from build123d import *

# Parameters (mm, degrees)
F0_R     = 12.7
F1_DEPTH = 30.1625
F2_W     = 28.956
F2_H     = 22.3266
F2_R     = 6.35
F3_DEPTH = 44.705
F5_DEPTH = 19.05
F7_DEPTH = 19.05
F8_R     = 3.302
F9_R     = 7.874
F10_R    = 3.302
F11_R    = 5.08


with BuildPart() as f1:
    # F0 (on Front) → F1 (new body, symmetric)
    with BuildSketch(Plane.XZ):
        with BuildLine():
            Line((-85.9282, -11.176), (108.2802, -11.176))
            Line((108.2802, -11.176), (108.2802, 11.176))
            Line((108.2802, 11.176), (-63.5762, 11.176))
            ThreePointArc((-63.5762, 11.176), (-101.733451, 26.981251), (-85.9282, -11.176))
        make_face()
        with Locations((-85.9282, 11.176)):
            Circle(F0_R, mode=Mode.SUBTRACT)
    extrude(amount=F1_DEPTH, both=True)

    # F2 (on face) → F3 (cut, through all)
    with BuildSketch(Plane(origin=(0, 0, -11.176), x_dir=(1, 0, 0), z_dir=(0, 0, -1))):
        with Locations((-100.4062, 0)):
            Rectangle(F2_W, F2_H)
        with Locations((69.4182, -7.8105)):
            Circle(F2_R)
        with Locations((-71.4502, 0)):
            Rectangle(F2_W, F2_H)
    extrude(amount=-F3_DEPTH, mode=Mode.SUBTRACT)

    # F4 (on face) → F5 (cut)
    with BuildSketch(Plane.XZ.offset(30.1625)):
        Polygon((31.3182, -11.176), (31.3182, 11.176), (-0.0762, 11.176), (5.9182, -11.176), align=None)
    extrude(amount=-F5_DEPTH, mode=Mode.SUBTRACT)

    # F6 (on face) → F7 (join)
    with BuildSketch(Plane.XZ.offset(30.1625)):
        with BuildLine():
            Line((31.3182, 9.144), (45.1104, 9.144))
            Line((45.1104, 9.144), (64.1604, 9.144))
            Line((64.1604, 9.144), (64.1604, 45.974))
            Line((64.1604, 45.974), (45.1104, 45.974))
            ThreePointArc((45.1104, 45.974), (41.536215, 27.258358), (31.3182, 11.176))
            Line((31.3182, 11.176), (31.3182, 9.144))
        make_face()
    extrude(amount=-F7_DEPTH)

    # F8
    f8_edges = [f1.edges().sort_by_distance(p)[0] for p in [
        (-63.5762, -20.6629, 11.176),
        (-63.5762, 20.6629, 11.176),
    ]]
    fillet(f8_edges, radius=F8_R)

    # F9
    f9_edges = [f1.edges().sort_by_distance(p)[0] for p in [
        (108.2802, 0, 11.176),
    ]]
    fillet(f9_edges, radius=F9_R)

    # F10
    f10_edges = [f1.edges().sort_by_distance(p)[0] for p in [
        (64.1604, -20.6375, 11.176),
    ]]
    fillet(f10_edges, radius=F10_R)

    # F11
    f11_edges = [f1.edges().sort_by_distance(p)[0] for p in [
        (64.1604, -20.6375, 45.974),
    ]]
    fillet(f11_edges, radius=F11_R)


solid = f1.part
Source: CAD feature listing. Evaluate the final solid. Frame: model axes, mm. A direction names the side the tool comes from. Give positions to 0.01 mm unless a question says otherwise; leave off trailing zeros. Write each loop counter-clockwise with the first axis right and the second up, starting at its lowest first coordinate (ties: lowest second). Pieces come first, ordered by that corner, then holes. Notation, with made-up numbers: M 27.25,21 L 60.25,21 A21 cw 60.25,32 Z; hole C 9,-8 d3. An arc over 180 degrees is marked long. Return JSON: item names as keys, results as strings. Group by question number.
1) Draft query along X for faces 1 (the face through (31.318, -21, 0)), 2 (the face through (15, -11.112, 0)), 3 (the face through (64.16, -21, 28)), 4 (the face through (-102.2, 20.5, 26.5)). Return one class per face: released by +X, released by -X, zero draft, split by the parting line, or undercut.
2) Cut plane B-B, the plane z = 17.5. Output: boundary loops of the cut face in (x, y), then the cut area to 3 significant figures.
3) Cut plane D-D, the plane y = 4. Output: boundary loops of the cut face in (x, z), then the cut area to 3 significant figures.
4) Set-up query: faces 5 (the face through (21, 6, 11.176)), 6 (the face through (-56.972, 0, 0)), 7 (the face through (53, -11.112, 29)). Return all of +Z, -Z, +X, -X, +Y, -Y with unobstructed straight access to the full face (end or side cutting, diameter ignored); none if empty.
5) First-contact query: pin 1 Ø5 at (y, z) = (11.5, 15.5) entering from -X; pin 2 Ø1.5 at (x, y) = (-25.5, 3) entering from +Z; pin 3 Ø18 at (y, z) = (-2, -4.5) entering from -X. Flat tips, straight axial feed; report the tip coordinate or a pass-through.
6) Ray query, L1, parallel to Y at x = -92.5, z = -4; L2, parallel to X at y = -15, z = -0.5; L3, parallel to Z at x = 50.5, y = 16. Return the intervals inside material, ascending.
7) Cut plane A-A, the plane y = 23. Output: boundary loops of the cut face in (x, z).
8) Cut plane C-C, the plane x = 49.5. Output: boundary loops of the cut face in (y, z), then the cut area to 3 significant figures.
Data:
{
 "1": {"face 1": "undercut", "face 2": "undercut", "face 3": "released by +X", "face 4": "split by the parting line"},
 "2": {"outline": "M -107.37,-30.16 L -96.94,-30.16 L -96.94,-11.16 L -107.37,-11.16 Z; M -107.37,11.16 L -96.94,11.16 L -96.94,30.16 L -107.37,30.16 Z; M -74.91,-30.16 L -64.49,-30.16 L -64.49,-11.16 L -74.91,-11.16 Z; M -74.91,11.16 L -64.49,11.16 L -64.49,30.16 L -74.91,30.16 Z; M 36.38,-30.16 L 64.16,-30.16 L 64.16,-11.11 L 36.38,-11.11 Z", "area": "1,320 mm²"},
 "3": {"outline": "M -56.97,-11.18 L 64.34,-11.18 L 64.34,11.18 L -56.97,11.18 Z; M 74.5,-11.18 L 108.28,-11.18 L 108.28,3.3 A7.87 ccw 100.41,11.18 L 74.5,11.18 Z", "area": "3,450 mm²"},
 "4": {"face 5": "+Z, +Y", "face 6": "+Z, -Z, -X", "face 7": "+Z, +X, -X, +Y"},
 "5": {"pin 1": "stops at x = -108.21", "pin 2": "stops at z = 11.18", "pin 3": "stops at x = -56.97"},
 "6": {"L1": "y = -30.16 to -11.16, 11.16 to 30.16", "L2": "x = -104.99 to -90.92, -80.93 to 3.06, 31.32 to 108.28", "L3": "z = -11.18 to 11.18"},
 "7": {"outline": "M -85.93,-11.18 L 108.28,-11.18 L 108.28,3.3 A7.87 ccw 100.41,11.18 L -60.49,11.18 A3.3 cw -63.76,14.05 A22.35 ccw long Z; hole C -85.93,11.18 d25.4"},
 "8": {"outline": "M -30.16,-11.18 L 30.16,-11.18 L 30.16,11.18 L -11.11,11.18 L -11.11,45.97 L -30.16,45.97 Z", "area": "2,010 mm²"}
}
